```python
from build123d import *

# Parameters (mm, degrees)
SKETCH_1_R          = 5.75
EXTRUDE_1_DEPTH     = 90
SKETCH_2_W          = 40
SKETCH_2_H          = 20
EXTRUDE_2_DEPTH     = 25
SKETCH_3_W          = 20.5
SKETCH_3_H          = 1
CUT_EXTRUDE_1_DEPTH = 20
FILLET_1_R          = 3


with BuildPart() as part:
    # 草图1 → 凸台-拉伸1 (new body)
    with BuildSketch(Plane(origin=(0, 0, 0), x_dir=(1, 0, 0), z_dir=(0, 1, 0))):
        with Locations(Location((0, 0, 0), (0, 0, 90))):
            Circle(SKETCH_1_R)
    extrude(amount=EXTRUDE_1_DEPTH)

    # 草图2 → 凸台-拉伸2 (add)
    with BuildSketch(Plane(origin=(0, 90, 0), x_dir=(1, 0, 0), z_dir=(0, 1, 0))):
        Rectangle(SKETCH_2_W, SKETCH_2_H)
    extrude(amount=EXTRUDE_2_DEPTH)

    # 草图3 → 切除-拉伸1 (cut)
    with BuildSketch(Plane(origin=(0, 115, 0), x_dir=(1, 0, 0), z_dir=(0, 1, 0))):
        Rectangle(SKETCH_3_W, SKETCH_3_H)
    extrude(amount=-CUT_EXTRUDE_1_DEPTH, mode=Mode.SUBTRACT)

    # 圆角1
    fillet_1_edges = [part.edges().sort_by_distance(p)[0] for p in [
        (20, 90, 0),
        (20, 102.5, 10),
        (0, 90, -10),
        (20, 102.5, -10),
        (-20, 90, 0),
        (-20, 102.5, -10),
        (0, 90, 10),
        (-20, 102.5, 10),
        (20, 115, 0),
        (0, 115, -10),
        (-20, 115, 0),
        (0, 115, 10),
    ]]
    fillet(fillet_1_edges, radius=FILLET_1_R)


solid = part.part
```
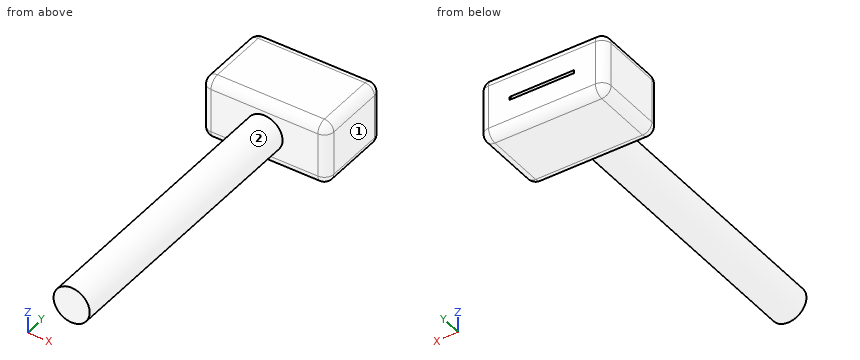
Read the model definition and answer for the solid it produces. Units are mm, in the model's axes. Face numbers are marked on the shaded views. A direction names the side the tool comes from. Round coordinates to 2 decimals unless told otherwise and drop trailing zeros. Loops run counter-clockwise (first coordinate to the right, second up) from the corner with the lowest first, then second, coordinate; pieces in that order, holes last. Notation, with made-up numbers: (-20.5, 5) -> (13.5, 5) arc R13 ccw to (13.5, 30) -> close; hole circle Ø1 at (45.5, -3). An arc over 180 degrees is marked (long way). One line per item, written item: value.
1) Flat-ended cylindrical pins translate along their axes: P1, Ø12, axis at x = -15, y = 85, coming from the -Z side; P2, Ø0.5, axis at x = -1.5, z = 0, coming from the +Y side; P3, Ø5, axis at x = 6, z = 7, coming from the -Y side. Find the tip coordinate at first contact, or state that the pin passes through.
Answer list:
P1: stops at z = -9.24
P2: stops at y = 95
P3: stops at y = 90
2) Consider L1, parallel to Z at x = -0.5, y = 101.5; L2, parallel to Y at x = -2, z = 6; L3, parallel to Y at x = 4.5, z = 0.25. Determine where each line is inside the solid, lowest interval first. Write a range as [from, to].
Answer list:
L1: z = [-10, -0.5], [0.5, 10]
L2: y = [90, 115]
L3: y = [0, 95]
3) A cutting plane is placed at A-A (y = 98). Determine the outline of the cut face in (x, z), and give its area (3 significant figures).
Answer list:
outline: (-20, -7) arc R3 ccw to (-17, -10) -> (17, -10) arc R3 ccw to (20, -7) -> (20, 7) arc R3 ccw to (17, 10) -> (-17, 10) arc R3 ccw to (-20, 7) -> close; hole (-10.25, -0.5) -> (10.25, -0.5) -> (10.25, 0.5) -> (-10.25, 0.5) -> close
area: 772 mm²
4) A cutting plane is placed at B-B (x = 0). Determine the outline of the cut face in (y, z).
Answer list:
outline: (0, -5.75) -> (90, -5.75) -> (90, -7) arc R3 ccw to (93, -10) -> (112, -10) arc R3 ccw to (115, -7) -> (115, -0.5) -> (95, -0.5) -> (95, 0.5) -> (115, 0.5) -> (115, 7) arc R3 ccw to (112, 10) -> (93, 10) arc R3 ccw to (90, 7) -> (90, 5.75) -> (0, 5.75) -> close
5) A cutting plane is placed at D-D (x = 9). Determine the outline of the cut face in (y, z).
Answer list:
outline: (90, -7) arc R3 ccw to (93, -10) -> (112, -10) arc R3 ccw to (115, -7) -> (115, -0.5) -> (95, -0.5) -> (95, 0.5) -> (115, 0.5) -> (115, 7) arc R3 ccw to (112, 10) -> (93, 10) arc R3 ccw to (90, 7) -> close
6) For the marked faces 1 and 2, determine the directions among +Z, -Z, +X, -X, +Y, -Y from which every point of the face is accessible in a straight line to the end or side of a thin tool.
Answer list:
face 1: +Z, -Z, +X, +Y, -Y
face 2: -Y
7) A cutting plane is placed at C-C (z = -8.25). Determine the outline of the cut face in (x, y), and give its area (3 significant figures).
Answer list:
outline: (-19.73, 93) arc R2.73 ccw to (-17, 90.27) -> (17, 90.27) arc R2.73 ccw to (19.73, 93) -> (19.73, 112) arc R2.73 ccw to (17, 114.73) -> (-17, 114.73) arc R2.73 ccw to (-19.73, 112) -> close
area: 958 mm²
